```python
from build123d import *

# Parameters (mm, degrees)
SKETCH_1_W          = 106
SKETCH_1_H          = 60
EXTRUDE_1_DEPTH     = 3
SKETCH_2_R          = 1.5
CUT_EXTRUDE_1_DEPTH = 10
FILLET_1_R          = 2


with BuildPart() as part:
    # 草图1 → 凸台-拉伸1 (new body)
    with BuildSketch(Plane(origin=(0, 0, 0), x_dir=(1, 0, 0), z_dir=(0, 1, 0))):
        Rectangle(SKETCH_1_W, SKETCH_1_H)
    extrude(amount=EXTRUDE_1_DEPTH)

    # 草图2 → 切除-拉伸1 (cut)
    with BuildSketch(Plane(origin=(0, 3, 0), x_dir=(1, 0, 0), z_dir=(0, 1, 0))):
        with Locations(Location((-48, 25, 0), (0, 0, 270))):
            Circle(SKETCH_2_R)
        with Locations(Location((-48, 0, 0), (0, 0, 270))):
            Circle(SKETCH_2_R)
        with Locations(Location((-48, -25, 0), (0, 0, 270))):
            Circle(SKETCH_2_R)
        with Locations(Location((48, -25, 0), (0, 0, 270))):
            Circle(SKETCH_2_R)
        with Locations(Location((48, 0, 0), (0, 0, 270))):
            Circle(SKETCH_2_R)
        with Locations(Location((48, 25, 0), (0, 0, 270))):
            Circle(SKETCH_2_R)
    extrude(amount=-CUT_EXTRUDE_1_DEPTH, mode=Mode.SUBTRACT)

    # 圆角1
    fillet_1_edges = [part.edges().sort_by_distance(p)[0] for p in [
        (53, 1.5, 30),
        (-53, 1.5, 30),
        (-53, 1.5, -30),
        (53, 1.5, -30),
    ]]
    fillet(fillet_1_edges, radius=FILLET_1_R)


solid = part.part
```
Verification items for the finished model (mm, model axes). Give positions to 0.01 mm unless a question says otherwise; leave off trailing zeros. Write each loop counter-clockwise with the first axis right and the second up, starting at its lowest first coordinate (ties: lowest second). Pieces come first, ordered by that corner, then holes. Notation, with made-up numbers: (-11.5, 72.25) - (20.5, 72.25) arc R21 cw to (20.5, 96.25) - close; hole circle Ø8 at (39.25, 43.25). An arc over 180 degrees is marked (long way). Put each result on its own line as item: value.
Q1. Mould release check, pull along Z, two halves, no side actions. Record for faces 1 (the face through (52.4, 1.52, 29.43)), 2 (the face through (-49.464, 1.521, -0.325)), 3 (the face through (53, 1, 0)): released by +Z, released by -Z, zero draft, split by the parting line, or undercut.
Result:
face 1: released by +Z
face 2: undercut
face 3: zero draft
Q2. Section check A-A on x = -48. Record the cut outline in (y, z).
Result:
outline: (0, -30) - (3, -30) - (3, -26.5) - (0, -26.5) - close; (0, -23.5) - (3, -23.5) - (3, -1.5) - (0, -1.5) - close; (0, 1.5) - (3, 1.5) - (3, 23.5) - (0, 23.5) - close; (0, 26.5) - (3, 26.5) - (3, 30) - (0, 30) - close
Q3. Scan lines: probe 1 along X at (y, z) = (1.1, -25); probe 2 along Z at (x, y) = (-47, 2.1). Record each from-to range of solid material in increasing order. Write a range as from..to.
Result:
probe 1: -53..-49.5, -46.5..46.5, 49.5..53
probe 2: -30..-26.12, -23.88..-1.12, 1.12..23.88, 26.12..30
Q4. Section check B-B on z = 25. Record the cut outline in (x, y).
Result:
outline: (-53, 0) - (-49.5, 0) - (-49.5, 3) - (-53, 3) - close; (-46.5, 0) - (46.5, 0) - (46.5, 3) - (-46.5, 3) - close; (49.5, 0) - (53, 0) - (53, 3) - (49.5, 3) - close
Q5. Section check C-C on z = -0.5. Record the cut outline in (x, y), and give its area (3 significant figures).
Result:
outline: (-53, 0) - (-49.41, 0) - (-49.41, 3) - (-53, 3) - close; (-46.59, 0) - (46.59, 0) - (46.59, 3) - (-46.59, 3) - close; (49.41, 0) - (53, 0) - (53, 3) - (49.41, 3) - close
area: 301 mm2
